Autodesk Fusion 360 part; units mm, degrees
sketch "Sketch1" plane through (0, 0, 0) normal (0, 1, 0) x (1, 0, 0)
  line L0 (0, 0) -> (42, 0)
  line L1 (0, 0) -> (0, -6)
  line L2 (42, 0) -> (42, -6)
  line L3 (42, -6) -> (31, -6)
  line L4 (31, -6) -> (31, -37.5)
  line L5 (0, -6) -> (11, -6)
  line L6 (11, -6) -> (11, -37.5)
  line L7 (11, -37.5) -> (31, -37.5)
  dimension "d1" = 42
  dimension "d2" = 6
  dimension "d3" = 6
  dimension "d7" = 11
  dimension "d8" = 31.5
  dimension "d9" = 11
  dimension "d10" = 31.5
extrude "Extrude1" add sketch "Sketch1" along normal blind 14
sketch "Sketch2" plane through (0, 0, 0) normal (0, -1, 0) x (1, 0, 0)
  line L0 (0, 6) -> (0, 0)
  line L1 (0, 0) -> (42, 0)
  line L2 (42, 0) -> (42, 6)
  line L3 (42, 6) -> (31, 6)
  line L4 (31, 6) -> (31, 37.5)
  line L5 (31, 37.5) -> (11, 37.5)
  line L6 (11, 37.5) -> (11, 6)
  line L7 (11, 6) -> (0, 6)
  line L8 (0, 0) -> (21, 0)
  line L9 (21, 0) -> (21, 23)
  circle A0 centre (21, 23) radius 6
  line L10 (21, 37.5) -> (23, 37.5)
  line L11 (21, 37.5) -> (19, 37.5)
  line L12 (19, 37.5) -> (19, 28.6569)
  line L13 (23, 37.5) -> (23, 28.6569)
  dimension "d13" = 23
  dimension "d14" = 12
  dimension "d15" = 2
  dimension "d16" = 2
extrude "Extrude2" cut sketch "Sketch2" against normal blind 49.568 contours A0 | L5 A0 L10 L11 L12 L13
sketch "Sketch3" plane through (0, 0, 6) normal (0, 0, 1) x (-1, 0, 0)
  line L0 (0, 0) -> (-11, 0)
  line L1 (-11, 0) -> (-11, -14)
  line L2 (-11, -14) -> (0, -14)
  line L3 (0, -14) -> (0, 0)
  line L4 (-5.5, -14) -> (-5.5, 0)
  line L5 (0, -7) -> (-11, -7)
  circle A0 centre (-5.5, -7) radius 2.75
  dimension "d19" = 5.5
extrude "Extrude3" cut sketch "Sketch3" against normal blind 15.501 contours L4 L5 A0 | L4 L5 A0 | L4 L5 A0 | L4 L5 A0
sketch "Sketch4" plane through (0, 0, 6) normal (0, 0, 1) x (-1, 0, 0)
  line L0 (-31, 0) -> (-42, 0)
  line L1 (-42, 0) -> (-42, -14)
  line L2 (-42, -14) -> (-31, -14)
  line L3 (-31, -14) -> (-31, 0)
  circle A0 centre (-36.5, -7) radius 2.75
  dimension "d22" = 5.5
extrude "Extrude4" cut sketch "Sketch4" against normal blind 36.862 contours A0
Geometry: final body of the model. Coordinates: model frame, mm. A direction names the side the tool comes from. Give positions to 0.01 mm unless a question says otherwise; leave off trailing zeros. Loops run counter-clockwise (first coordinate to the right, second up) from the corner with the lowest first, then second, coordinate; pieces in that order, holes last. Notation, with made-up numbers: (26.5, 41.5) -> (35.5, 41.5) arc R31 ccw to (35.5, 71.5) -> close; hole circle Ø8 at (6, -37). An arc over 180 degrees is marked (long way). Return JSON: item names as keys, results as strings.
Item 1: Section C-C, the plane y = 7. Output: boundary loops of the cut face in (x, z), plus the area to 3 significant figures.
Filled in:
{"outline": "(0, 0) -> (2.75, 0) -> (2.75, 6) -> (0, 6) -> close; (8.25, 0) -> (33.75, 0) -> (33.75, 6) -> (31, 6) -> (31, 37.5) -> (23, 37.5) -> (23, 28.66) arc R6 cw (long way) to (19, 28.66) -> (19, 37.5) -> (11, 37.5) -> (11, 6) -> (8.25, 6) -> close; (39.25, 0) -> (42, 0) -> (42, 6) -> (39.25, 6) -> close", "area": "668 mm^2"}
Item 2: Access query for faces 4 (the flat face through (11, 7, 22)), 5 (the flat face through (39, 8.5, 6)), 6 (the flat face through (19, 7, 33)). Directions: +Z, -Z, +X, -X, +Y, -Y. A direction counts if a zero-diameter tool reaches every point of the face in a straight line with its end or side. Return the directions, or none.
Filled in:
{"face 4": "+Z, -X, +Y, -Y", "face 5": "+Z, +X, +Y, -Y", "face 6": "+Z, +Y, -Y"}
Item 3: Mould query, pull axis X, two halves, no side actions, for faces 1 (the flat face through (27, 7, 37.5)), 2 (the flat face through (23, 7, 33)), 3 (the flat face through (42, 7, 3)). Classes: released by +X, released by -X, zero draft, split by the parting line, or undercut.
Filled in:
{"face 1": "zero draft", "face 2": "undercut", "face 3": "released by +X"}
Item 4: Section A-A, the plane x = 36.5. Output: boundary loops of the cut face in (y, z), plus the area to 3 significant figures.
Filled in:
{"outline": "(0, 0) -> (4.25, 0) -> (4.25, 6) -> (0, 6) -> close; (9.75, 0) -> (14, 0) -> (14, 6) -> (9.75, 6) -> close", "area": "51.0 mm^2"}
Item 5: Section D-D, the plane z = 8.5. Output: boundary loops of the cut face in (x, y).
Filled in:
{"outline": "(11, 0) -> (31, 0) -> (31, 14) -> (11, 14) -> close"}
Item 6: Section B-B, the plane z = 23. Output: boundary loops of the cut face in (x, y).
Filled in:
{"outline": "(11, 0) -> (15, 0) -> (15, 14) -> (11, 14) -> close; (27, 0) -> (31, 0) -> (31, 14) -> (27, 14) -> close"}
Item 7: Pin query (flat end, axial travel): P1, Ø1, axis at y = 8, z = 31, coming from the +X side; P2, Ø1.5, axis at y = 1.5, z = 27.5, coming from the -X side; P3, Ø5.5, axis at x = 37.5, y = 6.5, coming from the +Z side; P4, Ø5, axis at x = 36.5, y = 7, coming from the +Z side. Return the tip coordinate at first contact, or that it passes through.
Filled in:
{"P1": "x = 31", "P2": "x = 11", "P3": "z = 6", "P4": "through"}
Item 8: Line query: line 1 (X direction, y = 7, z = 2.35); line 2 (X direction, y = 5.25, z = 33); line 3 (Z direction, x = 8, y = 5). Output: solid intervals per line, ascending.
Filled in:
{"line 1": "0 to 2.75, 8.25 to 33.75, 39.25 to 42", "line 2": "11 to 19, 23 to 31", "line 3": "0 to 6"}
